```python
from build123d import *

# Parameters (mm, degrees)
F0_W      = 76.2
F0_H      = 76.2
F1_DEPTH  = 25.4
F1_FACE_W = 76.2
F1_FACE_H = 76.2
F2_DEPTH  = 32.766
F3_W      = 25.4
F3_H      = 25.4
F4_DEPTH  = 12.7
F5_R      = 12.7
F7_DEPTH  = 25.4


with BuildPart() as f1:
    # F0 (on Front) → F1 (new body)
    with BuildSketch(Plane.XZ):
        with Locations((-89.903427, 73.106664)):
            Rectangle(F0_W, F0_H)
    extrude(amount=F1_DEPTH)

    # F1_face (on face) → F2 (join)
    with BuildSketch(Plane(origin=(-89.903427, -25.4, 73.106664), x_dir=(1, 0, 0), z_dir=(0, -1, 0))):
        Rectangle(F1_FACE_W, F1_FACE_H)
    extrude(amount=F2_DEPTH)

    # F3 (on face) → F4 (join)
    with BuildSketch(Plane.XZ.offset(58.166)):
        with Locations((-89.903427, 73.106664)):
            Rectangle(F3_W, F3_H)
    extrude(amount=F4_DEPTH)

    # F5 (on face) → F7 (join)
    with BuildSketch(Plane.YZ.offset(-51.803427)):
        with Locations((-38.1, 73.106664)):
            Circle(F5_R)
    extrude(amount=F7_DEPTH)


solid = f1.part
```
The model under review builds one solid part; all positions refer to its coordinate system, in mm. A direction names the side the tool comes from. Give positions to 0.01 mm unless a question says otherwise; leave off trailing zeros. Loops run counter-clockwise (first coordinate to the right, second up) from the corner with the lowest first, then second, coordinate; pieces in that order, holes last. Notation, with made-up numbers: (-2, 65.5) - (29, 65.5) arc R24 cw to (29, 96.5) - close; hole circle Ø9 at (43, 89.5). An arc over 180 degrees is marked (long way). Answer as a JSON object with one key per item and string values.
Q1. Add section A-A on x = -80. State the section outline as (y, z) points, plus the area to 3 significant figures.
Worked out:
{"outline": "(-70.87, 60.41) - (-58.17, 60.41) - (-58.17, 35.01) - (0, 35.01) - (0, 111.21) - (-58.17, 111.21) - (-58.17, 85.81) - (-70.87, 85.81) - close", "area": "4,750 mm^2"}
Q2. For faces 1 (the flat face through (-90, -64, 60.407)), 2 (the flat face through (-102.603, -64, 73)), 3 (the flat face through (-90, -64, 85.807)), list the 3-axis set-ups (+Z, -Z, +X, -X, +Y, -Y) from which the entire face can be reached by the end or side of a thin tool; tool diameter is ignored.
Worked out:
{"face 1": "-Z, +X, -X, -Y", "face 2": "+Z, -Z, -X, -Y", "face 3": "+Z, +X, -X, -Y"}
Q3. Add section C-C on z = 95. State the section outline as (x, y) points, plus the area to 3 significant figures.
Worked out:
{"outline": "(-128, -58.17) - (-51.8, -58.17) - (-51.8, 0) - (-128, 0) - close", "area": "4,430 mm^2"}
Q4. Add section D-D on y = -13. State the section outline as (x, z) points.
Worked out:
{"outline": "(-128, 35.01) - (-51.8, 35.01) - (-51.8, 111.21) - (-128, 111.21) - close"}
Q5. Add section B-B on y = -38.1. State the section outline as (x, z) points, plus the area to 3 significant figures.
Worked out:
{"outline": "(-128, 35.01) - (-51.8, 35.01) - (-51.8, 60.41) - (-26.4, 60.41) - (-26.4, 85.81) - (-51.8, 85.81) - (-51.8, 111.21) - (-128, 111.21) - close", "area": "6,450 mm^2"}
Q6. Insertion check: pin 1 (3 mm diameter, centred on y = -15, z = 84, fed in from +X); pin 2 (4 mm diameter, centred on x = -47.5, z = 84, fed in from +Y); pin 3 (10 mm diameter, centred on y = -64.5, z = 76, fed in from +X). Each pin has a flat end and moves straight along its axis. Give the tip position at first contact, or say it passes through.
Worked out:
{"pin 1": "stops at x = -51.8", "pin 2": "stops at y = -29.03", "pin 3": "stops at x = -77.2"}
Q7. To check wall thickness, follow line 1 along Y through (x, z) = (-78, 52); line 2 along X through (y, z) = (-18.5, 83); line 3 along Z through (x, y) = (-89, -62.5). State the ranges of each line that lie inside material, in increasing order.
Worked out:
{"line 1": "y = -58.17 to 0", "line 2": "x = -128 to -51.8", "line 3": "z = 60.41 to 85.81"}
